For this review, use the dimensioned drawing (mm, ordinates from the lowest corner) and the shaded views. A direction names the side the tool comes from. Coordinates: 2 decimals unless noted, no trailing zeros. Loops run counter-clockwise (first coordinate to the right, second up) from the corner with the lowest first, then second, coordinate; pieces in that order, holes last. Notation, with made-up numbers: (26, 87.5) - (51, 87.5) arc R25 cw to (51, 101.5) - close; hole circle Ø8 at (-31.5, 72.25). An arc over 180 degrees is marked (long way). Answer in a Markdown table with one row per item. Add a question column.
(1) The part is to be moulded in two halves that separate along X. For the marked faces 3, 4 and 5, say which applies: released by +X, released by -X, zero draft, split by the parting line, or undercut.
(2) We need section C-C, the plane y = 28. Write out the cut boundary in (x, z).
(3) To check wall thickness, follow L1, parallel to X at y = 14.5, z = 15.25; L2, parallel to Z at x = 4.25, y = 33; L3, parallel to Y at x = 3.25, z = 3.75. State the ranges of each line that lie inside material, in increasing order. Write a range as [from, to].
(4) We need section A-A, the plane z = 5.5. Write out the cut boundary in (x, y).
(5) For the marked faces 1 and 2, list the 3-axis set-ups (+Z, -Z, +X, -X, +Y, -Y) from which the entire face can be reached by the end or side of a thin tool; tool diameter is ignored.
(6) Clearance check with flat-ended pins moving along their axes: pin 1 (12 mm diameter, centred on y = 28.5, z = 17.5, fed in from -X); pin 2 (2 mm diameter, centred on x = 12, z = 10.5, fed in from -Y); pin 3 (0.9 mm diameter, centred on x = 10, y = 1, fed in from +Z). State where each tip first meets the part, or that it passes through.
(7) We need section B-B, the plane x = 17.5. Write out the cut boundary in (y, z), plus the area to 3 significant figures.
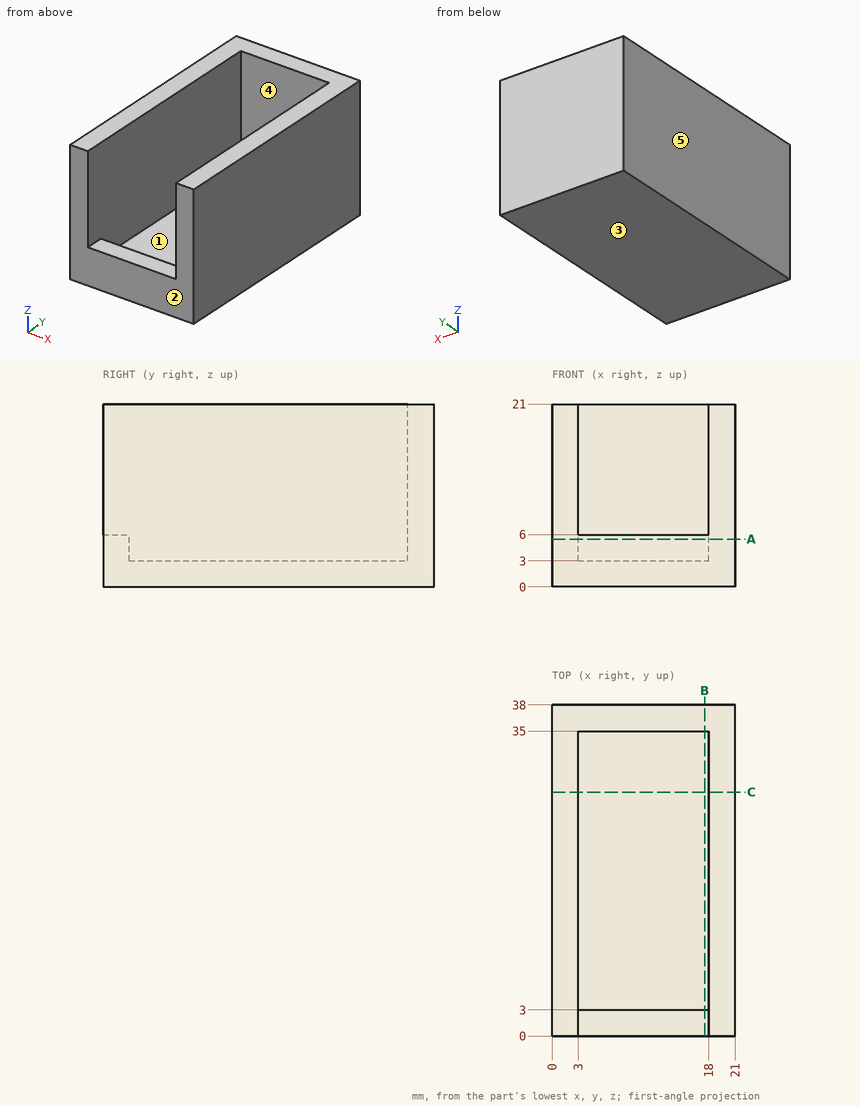
Responses:
| question | item | result |
|---|---|---|
| 1 | face 3 | zero draft |
| 1 | face 4 | undercut |
| 1 | face 5 | released by -X |
| 2 | outline | (0, 0) - (21, 0) - (21, 21) - (18, 21) - (18, 3) - (3, 3) - (3, 21) - (0, 21) - close |
| 3 | L1 | x = [0, 3], [18, 21] |
| 3 | L2 | z = [0, 3] |
| 3 | L3 | y = [0, 3], [35, 38] |
| 4 | outline | (0, 0) - (21, 0) - (21, 38) - (0, 38) - close; hole (3, 3) - (18, 3) - (18, 35) - (3, 35) - close |
| 5 | face 1 | +Z |
| 5 | face 2 | +Z, -Z, +X, -X, -Y |
| 6 | pin 1 | stops at x = 0 |
| 6 | pin 2 | stops at y = 35 |
| 6 | pin 3 | stops at z = 6 |
| 7 | outline | (0, 0) - (38, 0) - (38, 21) - (35, 21) - (35, 3) - (3, 3) - (3, 6) - (0, 6) - close |
| 7 | area | 177 mm2 |
